Part model, mm, in its own coordinate system. Face numbers are marked on the shaded views. A direction names the side the tool comes from. Give positions to 0.01 mm unless a question says otherwise; leave off trailing zeros. Order: outer loops, then holes, each group sorted by start corner. A loop starts at its lowest first (then second) coordinate and runs counter-clockwise, first axis right, second up. Notation, with made-up numbers: (-29.75, -28.75) - (-19.75, -28.75) arc R12 ccw to (-19.75, -15.75) - close; hole circle Ø6 at (78.25, 66). An arc over 180 degrees is marked (long way). One line per item, written item: value.
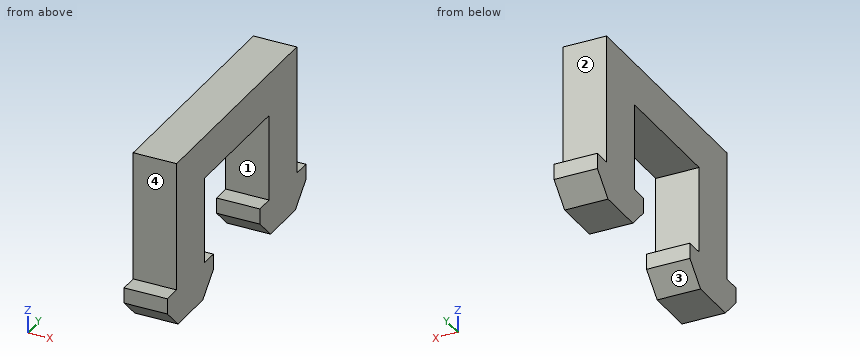
```python
from build123d import *

# Parameters (mm, degrees)
BOSS_EXTRUDE1_DEPTH = 5
SKETCH3_W           = 4.925645198
SKETCH3_H           = 33.799871634
BOSS_EXTRUDE2_DEPTH = 5
SKETCH4_W           = 4.925645198
SKETCH4_H           = 6.649871634
CUT_EXTRUDE1_DEPTH  = 37.492986368


with BuildPart() as part:
    # Sketch2 → Boss-Extrude1 (new body)
    with BuildSketch(Plane(origin=(0, 0, 0), x_dir=(0, 0, -1), z_dir=(1, 0, 0))):
        Polygon((-4.2, 3.125), (-14.2, 3.125), (-14.2, -3.125), (-4.2, -3.125), (-4.2, -5.2), (-2.4, -5.2), (0, -2.8), (0, 2.8), (-2.4, 5.2), (-4.2, 5.2), align=None)
    boss_extrude1 = extrude(amount=BOSS_EXTRUDE1_DEPTH)

    # Sketch3 → Boss-Extrude2 (add)
    with BuildSketch(Plane.ZY):
        with Locations((16.662822599, 13.774935817)):
            Rectangle(SKETCH3_W, SKETCH3_H)
    extrude(amount=-BOSS_EXTRUDE2_DEPTH)

    # Mirror2: Boss-Extrude1 across plane
    add(boss_extrude1.mirror(Plane.ZX.offset(10.45)))

    # Sketch4 → Cut-Extrude1 (cut, through all)
    with BuildSketch(Plane.ZY):
        with Locations((16.662822599, 27.349935817)):
            Rectangle(SKETCH4_W, SKETCH4_H)
    extrude(amount=-CUT_EXTRUDE1_DEPTH, mode=Mode.SUBTRACT)


solid = part.part
```
1) Which spindle directions (+Z, -Z, +X, -X, +Y, -Y) get a long thin tool onto all of the face, cutting with end or side? Do the marked faces 1, 2, 3 and 4. Say none if no direction does.
Outcome:
face 1: +X, -X
face 2: +Z, +X, -X, +Y
face 3: -Z, +X, -X
face 4: +Z, +X, -X, -Y
2) Cut at C-C, the plane x = 3.65. Give the cut face in (y, z) (3 decimals), then the cut area to 3 significant figures.
Outcome:
outline: (-5.2, 2.4) - (-2.8, 0) - (2.8, 0) - (5.2, 2.4) - (5.2, 4.2) - (3.125, 4.2) - (3.125, 14.2) - (17.775, 14.2) - (17.775, 4.2) - (15.7, 4.2) - (15.7, 2.4) - (18.1, 0) - (23.7, 0) - (26.1, 2.4) - (26.1, 4.2) - (24.025, 4.2) - (24.025, 19.126) - (-3.125, 19.126) - (-3.125, 4.2) - (-5.2, 4.2) - close
area: 335 mm^2
3) Drill centre lines: line 1 along Y through (x, z) = (3.6, 6.25) (3 decimals); line 2 along Y through (x, z) = (0.45, 4); line 3 along Y through (x, z) = (2.5, 16.5) (3 decimals). Where is each one in solid material? Low to high. Write a range as from..to.
Outcome:
line 1: y = -3.125..3.125, 17.775..24.025
line 2: y = -5.2..5.2, 15.7..26.1
line 3: y = -3.125..24.025
4) Cut at D-D, the plane z = 15.75. Give the cut face in (x, y) (3 decimals).
Outcome:
outline: (0, -3.125) - (5, -3.125) - (5, 24.025) - (0, 24.025) - close
5) Cut at A-A, the plane y = 4. Give the cut face in (x, z), then the cut area to 3 significant figures.
Outcome:
outline: (0, 1.2) - (5, 1.2) - (5, 4.2) - (0, 4.2) - close; (0, 14.2) - (5, 14.2) - (5, 19.13) - (0, 19.13) - close
area: 39.6 mm^2
6) Cut at B-B, the plane z = 8.5. Give the cut face in (x, y) (3 decimals).
Outcome:
outline: (0, -3.125) - (5, -3.125) - (5, 3.125) - (0, 3.125) - close; (0, 17.775) - (5, 17.775) - (5, 24.025) - (0, 24.025) - close
7) Pin check, flat tips, straight feed: pin 1 (3 mm diameter, centred on x = 0.5, z = 15.5, fed in from +Y) (3 decimals); pin 2 (1 mm diameter, centred on x = 3.5, y = 11, fed in from -Z); pin 3 (0.6 mm diameter, centred on x = 2.5, y = 25, fed in from +Z). Stop position of each tip, or through.
Outcome:
pin 1: stops at y = 24.025
pin 2: stops at z = 14.2
pin 3: stops at z = 4.2
